Verification items for the finished model (mm, model axes). A direction names the side the tool comes from. Round coordinates to 2 decimals unless told otherwise and drop trailing zeros. Write each loop counter-clockwise with the first axis right and the second up, starting at its lowest first coordinate (ties: lowest second). Pieces come first, ordered by that corner, then holes. Notation, with made-up numbers: (69.25, 3.25) - (81.25, 3.25) arc R20 ccw to (81.25, 42.25) - close; hole circle Ø11 at (37, 86). An arc over 180 degrees is marked (long way). Answer as a JSON object with one key per item and string values.
```python
from build123d import *

# Parameters (mm, degrees)
F0_R     = 6.35
F0_R_2   = 3.175
F1_DEPTH = 15.875
F3_DEPTH = 9.525
F4_W     = 3.175
F4_H     = 3.175
F6_R     = 1.58749


# Not quite as in the source:
# - a fillet or chamfer is up to 0.001 mm smaller than in the source, because OpenCascade refuses the exact size


with BuildPart() as f1:
    # F0 (on Top) → F1 (new body)
    with BuildSketch(Plane.XY):
        Circle(F0_R)
        Circle(F0_R_2, mode=Mode.SUBTRACT)
        Circle(F0_R_2)
    extrude(amount=F1_DEPTH)

    # F0 (on Top) → F3 (join)
    with BuildSketch(Plane.XY):
        Circle(F0_R_2)
    extrude(amount=-F3_DEPTH)

    # F4 (on Right) → F5 (revolve, cut)
    with BuildSketch(Plane.YZ):
        with Locations((4.7625, 4.7625)):
            Rectangle(F4_W, F4_H)
        with Locations((4.7625, 11.1125)):
            Rectangle(F4_W, F4_H)
    revolve(axis=Axis((0, 0, -0.284396112), (0, 0, 1)), mode=Mode.SUBTRACT)

    # F6 (radius 1.5875 in the source; OpenCascade refuses exactly that, so slightly less here)
    f6_edges = [f1.edges().sort_by_distance(p)[0] for p in [
        (0, -3.175, 3.175),
        (0, -3.175, 6.35),
        (0, -3.175, 9.525),
        (0, -3.175, 12.7),
    ]]
    fillet(f6_edges, radius=F6_R)


solid = f1.part
```
Q1. Section check D-D, the plane z = -4.25. Record the cut outline in (x, y) (3 decimals).
Geometry check:
{"outline": "circle Ø6.35 at (0, 0)"}
Q2. Section check C-C, the plane y = 5.5. Record the cut outline in (x, z) (3 decimals).
Geometry check:
{"outline": "(-3.174, 0) - (3.174, 0) - (3.174, 3.175) - (-3.174, 3.175) - close; (-3.174, 6.35) - (3.174, 6.35) - (3.174, 9.525) - (-3.174, 9.525) - close; (-3.174, 12.7) - (3.174, 12.7) - (3.174, 15.875) - (-3.174, 15.875) - close"}
Q3. Set-up check for faces 1 (the flat face through (-5, -1, 9.525)), 2 (the flat face through (-2, 3, 0)), 3 (the flat face through (0, 0, -9.525)): record each of +Z, -Z, +X, -X, +Y, -Y from which the full face is reachable in a straight line by a thin tool's end or side.
Geometry check:
{"face 1": "none", "face 2": "-Z", "face 3": "-Z, +X, -X, +Y, -Y"}
Q4. Material ranges on line 1 along Z through (x, y) = (-0.75, 5.5) (3 decimals); line 2 along Z through (x, y) = (-1.75, -3.75) (3 decimals); line 3 along Y through (x, z) = (-0.25, 8), recorded low to high. Write a range as [from, to].
Geometry check:
{"line 1": "z = [0, 3.175], [6.35, 9.525], [12.7, 15.875]", "line 2": "z = [0, 3.303], [6.222, 9.653], [12.572, 15.875]", "line 3": "y = [-6.35, 6.35]"}
Q5. Gauge pin test, flat ends, axial feed: P1, Ø1.5, axis at y = 0, z = 12.5, coming from the -X side; P2, Ø1.5, axis at y = -2.5, z = 10, coming from the -X side; P3, Ø1.5, axis at y = -4, z = 1.5, coming from the -X side; P4, Ø6, axis at x = 4.5, z = 10, coming from the -Y side. Record the tip position at first contact, or that the pin passes through.
Geometry check:
{"P1": "stops at x = -6.35", "P2": "stops at x = -6.05", "P3": "stops at x = -5.46", "P4": "stops at y = -6.16"}
